Read the model definition and answer for the solid it produces. Units are mm, in the model's axes. A direction names the side the tool comes from. Give positions to 0.01 mm unless a question says otherwise; leave off trailing zeros. Loops run counter-clockwise (first coordinate to the right, second up) from the corner with the lowest first, then second, coordinate; pieces in that order, holes last.
(1) Straight lines are drawn through the part: probe 1 along Z at (x, y) = (-26.9, 32); probe 2 along X at (y, z) = (0, 13.75); probe 3 along X at (y, z) = (44, 6.75). For each, find the intervals that lie inside material, in ascending order.
(2) Find section D-D, the plane z = 17.25. Write down the section's boundary in (x, y).
(3) Find section A-A, the plane z = 10. Write down the section's boundary in (x, y).
(4) Determine the mould class of faces 3 (the face through (16.214, 21.268, 9.868)), 4 (the face through (-27, 51.6, 0.2)), 5 (the face through (-21, -15, 0)) for opening direction X: pulls with the +X half, pulls with the -X half, needs draft (parallel to the pull), parting line crosses it, or undercut.
(5) Find section B-B, the plane y = 32. Write down the section's boundary in (x, z).
(6) Find section C-C, the plane x = 0. Write down the section's boundary in (y, z).
(7) Each of these flat-tipped pins is pushed along its axis until it touches: P1, Ø10, axis at y = 21, z = 15, coming from the +X side; P2, Ø10, axis at y = 30, z = 13.5, coming from the +X side; P3, Ø7, axis at y = 44, z = 10, coming from the +X side. Where does it stop, or does it pass through?
(8) Which of the six approach directions +Z, -Z, +X, -X, +Y, -Y give full straight-line access (tool end or side, diameter ignored) to faces 1 (the face through (-25, 25, 10)), 2 (the face through (10.357, -27.087, 9.868))?
```python
from build123d import *

# Parameters (mm, degrees)
PAD_DEPTH    = 20
SKETCH001_R  = 2.25
POCKET_DEPTH = 5
CHAMFER_SIZE = 0.6


with BuildPart() as part:
    # Sketch → Pad (new body)
    with BuildSketch(Plane.XY):
        with BuildLine():
            ThreePointArc((-25, 0), (9.567086, -23.096988), (17.67767, 17.67767))
            ThreePointArc((17.67767, 24.748737), (16.213203, 21.213203), (17.67767, 17.67767))
            ThreePointArc((20.506097, 21.92031), (20.506097, 24.748737), (17.67767, 24.748737))
            ThreePointArc((20.506097, 21.92031), (20.213203, 21.213203), (20.506097, 20.506097))
            ThreePointArc((-29, 0), (11.09782, -26.792506), (20.506097, 20.506097))
            Line((-29, 0), (-29, 50))
            ThreePointArc((-25, 50), (-27, 52), (-29, 50))
            Line((-25, 0), (-25, 50))
        make_face()
    extrude(amount=PAD_DEPTH)

    # Sketch001 (on Face3 of Pad) → Pocket (cut)
    with BuildSketch(Plane.YZ.offset(-25)):
        with Locations((44, 10)):
            Circle(SKETCH001_R)
        with Locations((32, 10)):
            Circle(SKETCH001_R)
    extrude(amount=-POCKET_DEPTH, mode=Mode.SUBTRACT)

    # Chamfer
    chamfer_edges = [part.edges().sort_by_distance(p)[0] for p in [
        (-25, 29.75, 10),
        (-25, 41.75, 10),
        (-29, 25, 20),
        (-27, 52, 20),
        (-25, 25, 20),
        (9.567086, -23.096988, 20),
        (16.213203, 21.213203, 20),
        (20.506097, 24.748737, 20),
        (20.213203, 21.213203, 20),
        (11.09782, -26.792506, 20),
        (-29, 25, 0),
        (-27, 52, 0),
        (-25, 25, 0),
        (9.567086, -23.096988, 0),
        (16.213203, 21.213203, 0),
        (20.506097, 24.748737, 0),
        (20.213203, 21.213203, 0),
        (11.09782, -26.792506, 0),
        (-29, 29.75, 10),
        (-29, 41.75, 10),
    ]]
    chamfer(chamfer_edges, length=CHAMFER_SIZE)


solid = part.part
```
Entries:
1. probe 1: z = 0 to 7.75, 12.25 to 20
1. probe 2: x = -29 to -25, 25 to 29
1. probe 3: x = -29 to -25
2. outline: (-29, 0) arc R29 ccw (long way) to (20.51, 20.51) arc R1 cw to (20.51, 21.92) arc R2 ccw to (17.68, 24.75) arc R5 ccw to (17.68, 17.68) arc R25 cw (long way) to (-25, 0) - (-25, 50) arc R2 ccw to (-29, 50) - close
3. outline: (-29, 0) arc R29 ccw (long way) to (20.51, 20.51) arc R1 cw to (20.51, 21.92) arc R2 ccw to (17.68, 24.75) arc R5 ccw to (17.68, 17.68) arc R25 cw (long way) to (-25, 0) - (-25, 29.15) - (-25.6, 29.75) - (-28.4, 29.75) - (-29, 29.15) - close; (-29, 34.85) - (-28.4, 34.25) - (-25.6, 34.25) - (-25, 34.85) - (-25, 41.15) - (-25.6, 41.75) - (-28.4, 41.75) - (-29, 41.15) - close; (-29, 46.85) - (-28.4, 46.25) - (-25.6, 46.25) - (-25, 46.85) - (-25, 50) arc R2 ccw to (-29, 50) - close
4. face 3: undercut
4. face 4: parting line crosses it
4. face 5: needs draft
5. outline: (-29, 0.6) - (-28.4, 0) - (-25.6, 0) - (-25, 0.6) - (-25, 7.15) - (-25.6, 7.75) - (-28.4, 7.75) - (-29, 7.15) - close; (-29, 12.85) - (-28.4, 12.25) - (-25.6, 12.25) - (-25, 12.85) - (-25, 19.4) - (-25.6, 20) - (-28.4, 20) - (-29, 19.4) - close
6. outline: (-29, 0.6) - (-28.4, 0) - (-25.6, 0) - (-25, 0.6) - (-25, 19.4) - (-25.6, 20) - (-28.4, 20) - (-29, 19.4) - close
7. P1: stops at x = 24.19
7. P2: stops at x = 20.2
7. P3: stops at x = -25
8. face 1: +Z, -Z, +Y
8. face 2: +Z, -Z
